```python
from build123d import *

# Parameters (mm, degrees)
BOSS_EXTRUDE1_DEPTH = 5
SKETCH2_W           = 118.181462396
SKETCH2_H           = 15.165331065
BOSS_EXTRUDE4_DEPTH = 47
SKETCH3_W           = 118.126380902
SKETCH3_H           = 20.616541225
BOSS_EXTRUDE5_DEPTH = 48
SKETCH4_W           = 8.296758782
SKETCH4_H           = 26.299414598
BOSS_EXTRUDE6_DEPTH = 30
CUT_EXTRUDE3_DEPTH  = 7
SKETCH6_W           = 2.21745904
SKETCH6_H           = 1.840019648
SKETCH6_W_2         = 2.568509623
SKETCH6_W_3         = 2.623522206
SKETCH6_H_2         = 1.802097087
BOSS_EXTRUDE7_DEPTH = 7


with BuildPart() as part:
    # Sketch1 → Boss-Extrude1 (new body)
    with BuildSketch(Plane(origin=(0, 0, 0), x_dir=(0, 0, -1), z_dir=(1, 0, 0))):
        with BuildLine():
            Line((10, 0), (131.29221645, 0))
            ThreePointArc((131.29221645, 0), (138.363284262, -2.928932188), (141.29221645, -10))
            Line((141.29221645, -10), (141.29221645, -104.488481637))
            ThreePointArc((141.29221645, -104.488481637), (138.363284262, -111.559549449), (131.29221645, -114.488481637))
            Line((131.29221645, -114.488481637), (10, -114.488481637))
            ThreePointArc((10, -114.488481637), (2.928932188, -111.559549449), (0, -104.488481637))
            Line((0, -104.488481637), (0, -10))
            ThreePointArc((0, -10), (2.928932188, -2.928932188), (10, 0))
        make_face()
    extrude(amount=BOSS_EXTRUDE1_DEPTH)

    # Sketch2 → Boss-Extrude4 (add)
    with BuildSketch(Plane(origin=(5, 0, 0), x_dir=(0, 0, -1), z_dir=(1, 0, 0))):
        with Locations((68.242208416, -80.606538465)):
            Rectangle(SKETCH2_W, SKETCH2_H)
    extrude(amount=BOSS_EXTRUDE4_DEPTH)

    # Sketch3 → Boss-Extrude5 (add)
    with BuildSketch(Plane(origin=(5, 0, 0), x_dir=(0, 0, -1), z_dir=(1, 0, 0))):
        with Locations((68.5485811, -98.427462894)):
            Rectangle(SKETCH3_W, SKETCH3_H)
    extrude(amount=BOSS_EXTRUDE5_DEPTH)

    # Sketch4 → Boss-Extrude6 (add)
    with BuildSketch(Plane(origin=(5, 0, 0), x_dir=(0, 0, -1), z_dir=(1, 0, 0))):
        with Locations((137.143837059, -88.907539255)):
            Rectangle(SKETCH4_W, SKETCH4_H)
    extrude(amount=BOSS_EXTRUDE6_DEPTH)

    # Sketch5 → Cut-Extrude3 (cut)
    with BuildSketch(Plane(origin=(0, 0, -141.29221645), x_dir=(-1, 0, 0), z_dir=(0, 0, -1))):
        Polygon((-25.464332728, -97.926181685), (-12.810425415, -97.926181685), (-8.73119877, -90.234247578), (-8.73119877, -80.275506322), (-31.116096198, -80.275506322), (-31.116096198, -91.525760494), align=None)
    extrude(amount=-CUT_EXTRUDE3_DEPTH, mode=Mode.SUBTRACT)

    # Sketch6 → Boss-Extrude7 (add)
    with BuildSketch(Plane(origin=(0, 0, -134.29221645), x_dir=(-1, 0, 0), z_dir=(0, 0, -1))):
        with Locations((-25.041507493, -87.601540864)):
            Rectangle(SKETCH6_W, SKETCH6_H)
        with Locations((-13.458219738, -87.601540864)):
            Rectangle(SKETCH6_W_2, SKETCH6_H)
        with Locations((-19.506551217, -92.8677498)):
            Rectangle(SKETCH6_W_3, SKETCH6_H_2)
    extrude(amount=BOSS_EXTRUDE7_DEPTH)


solid = part.part
```
Read the model definition and answer for the solid it produces. Units are mm, in the model's axes. A direction names the side the tool comes from. Give positions to 0.01 mm unless a question says otherwise; leave off trailing zeros. Write each loop counter-clockwise with the first axis right and the second up, starting at its lowest first coordinate (ties: lowest second). Pieces come first, ordered by that corner, then holes. Notation, with made-up numbers: (83.25, 47.25) -> (119.25, 47.25) arc R26 ccw to (119.25, 61.25) -> close; hole circle Ø3 at (68, 36.25). An arc over 180 degrees is marked (long way). Answer in a Markdown table with one row per item.
1) Straight lines are drawn through the part: line 1 (Z direction, x = 14, y = -83); line 2 (X direction, y = -46, z = -62.5); line 3 (Y direction, x = 29, z = -107.5). For each, find the intervals that lie inside material, in ascending order. Write a range as [from, to].
Results list:
| item | result |
|---|---|
| line 1 | [-134.29, -133], [-127.33, -9.15] |
| line 2 | [0, 5] |
| line 3 | [-108.74, -73.02] |
2) Section A-A on x = 33 is taken. Give the vertices of the cut face in (y, z), plus the area to 3 significant figures.
Results list:
| item | result |
|---|---|
| outline | (-108.74, -127.61) -> (-88.12, -127.61) -> (-88.12, -127.33) -> (-73.02, -127.33) -> (-73.02, -9.15) -> (-88.19, -9.15) -> (-88.19, -9.49) -> (-108.74, -9.49) -> close; (-102.06, -141.29) -> (-75.76, -141.29) -> (-75.76, -133) -> (-102.06, -133) -> close |
| area | 4,440 mm^2 |
3) Section C-C on y = -70 is taken. Give the vertices of the cut face in (x, z).
Results list:
| item | result |
|---|---|
| outline | (0, -141.29) -> (5, -141.29) -> (5, 0) -> (0, 0) -> close |
4) A tool of negligible diameter and unlimited length cuts with its end or side. For faces 1 (the flat face through (10.799, -94.134, -137.841)), 2 (the flat face through (28, -73.024, -67)), 3 (the flat face through (35, -89, -137)), 4 (the flat face through (20, -75.758, -137)), from which of +Z, -Z, +X, -X, +Y, -Y can it reach the whole face along a straight path? Write none if from no direction.
Results list:
| item | result |
|---|---|
| face 1 | -Z |
| face 2 | +Z, -Z, +X, +Y |
| face 3 | -Z, +X, +Y, -Y |
| face 4 | -Z, +X, +Y |
5) Section B-B on z = -121.5 is taken. Give the vertices of the cut face in (x, y).
Results list:
| item | result |
|---|---|
| outline | (0, -114.49) -> (5, -114.49) -> (5, -108.74) -> (53, -108.74) -> (53, -88.12) -> (52, -88.12) -> (52, -73.02) -> (5, -73.02) -> (5, 0) -> (0, 0) -> close |
6) Each of these flat-tipped pins is pushed along its axis until it touches: pin 1 Ø2 at (x, z) = (19, -37) entering from -Y; pin 2 Ø9 at (x, z) = (12.5, -137) entering from +Y; pin 3 Ø13 at (x, y) = (18, -93.5) entering from +Z. Where does it stop, or does it pass through?
Results list:
| item | result |
|---|---|
| pin 1 | y = -108.74 |
| pin 2 | y = -75.76 |
| pin 3 | z = -9.15 |
7) Determine the mould class of faces 5 (the cylindrical face through (2.46, -111.64, -3.01)), 6 (the flat face through (29, -99, -127.612)), 7 (the flat face through (20, -102.057, -137)), 8 (the flat face through (28, -81, -127.333)) for opening direction Z: released by +Z, released by -Z, zero draft, split by the parting line, or undercut.
Results list:
| item | result |
|---|---|
| face 5 | released by +Z |
| face 6 | undercut |
| face 7 | zero draft |
| face 8 | undercut |
